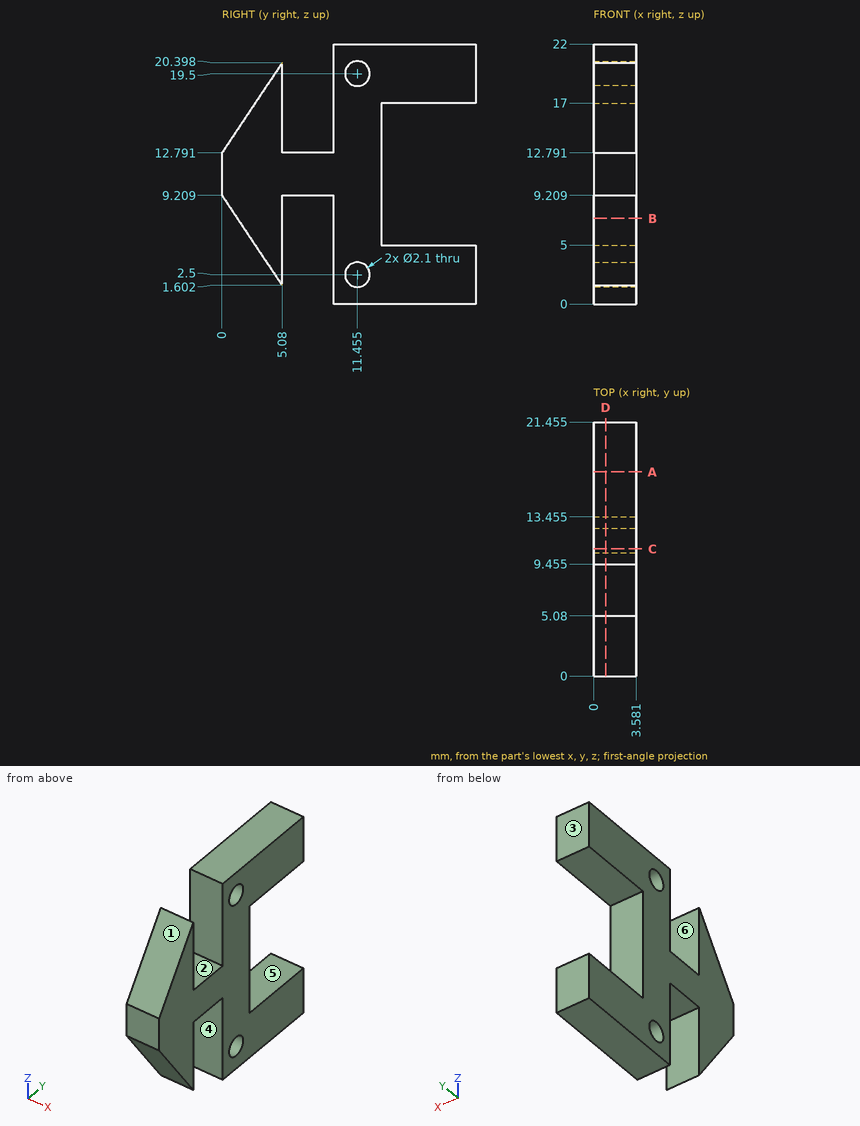
Answer from the drawing. Dimensions are ordinates in mm from the lowest x, y and z of the part. A direction names the side the tool comes from. Give positions to 0.01 mm unless a question says otherwise; leave off trailing zeros. Loops run counter-clockwise (first coordinate to the right, second up) from the corner with the lowest first, then second, coordinate; pieces in that order, holes last. Notation, with made-up numbers: (45.5, 52.25) -> (63.5, 52.25) arc R20 ccw to (63.5, 58.25) -> close; hole circle Ø4 at (-14.5, -32.5). An arc over 180 degrees is marked (long way). One line per question, with ' | ' between items. Start each with the question number.
1) Straight lines are drawn through the part: L1, parallel to Z at x = 1.45, y = 13.5; L2, parallel to Y at x = 1.75, z = 19.5 (1 decimal); L3, parallel to Z at x = 1.7, y = 5.75. For each, find the intervals that lie inside material, in ascending order.
2) Determine the mould class of the marked faces 1, 2 and 3 for opening direction Y: +Y half, -Y half, draft (parallel to the pull), parting line (faces both ways), or undercut.
3) Section B-B, the plane z = 7.25 is taken. Determine the outline of the cut face in (x, y) (1 decimal).
4) Section D-D, the plane x = 1 is taken. State how many separate pieces and enclosed holes the cut face has.
5) For the marked faces 4, 5 and 6, determine the directions among +Z, -Z, +X, -X, +Y, -Y from which every point of the face is accessible in a straight line to the end or side of a thin tool.
6) Section A-A, the plane y = 17.25 is taken. Determine the outline of the cut face in (x, z).
7) Each of these flat-tipped pins is pushed along its axis until it touches: pin 1 (2 mm diameter, centred on x = 2.5, z = 18, fed in from -Y); pin 2 (1.7 mm diameter, centred on y = 11.45, z = 2.5, fed in from -X); pin 3 (1.1 mm diameter, centred on x = 2, z = 12.5, fed in from +Y) (3 decimals); pin 4 (1.8 mm diameter, centred on x = 1.5, y = 7.5, fed in from +Z). Where does it stop, or does it pass through?
8) Section C-C, the plane y = 10.75 is taken. Determine the outline of the cut face in (x, z).
Resolved:
1) L1: 0 to 5, 17 to 22 | L2: 4.5 to 5.1, 9.5 to 10.4, 12.5 to 21.5 | L3: 9.21 to 12.79
2) face 1: -Y half | face 2: undercut | face 3: +Y half
3) outline: (0, 1.3) -> (3.6, 1.3) -> (3.6, 5.1) -> (0, 5.1) -> close; (0, 9.5) -> (3.6, 9.5) -> (3.6, 13.5) -> (0, 13.5) -> close
4) separate pieces: 1 | enclosed holes: 2
5) face 4: -Z, +X, -X | face 5: +X, -X, +Y | face 6: +Z, +X, -X
6) outline: (0, 0) -> (3.58, 0) -> (3.58, 5) -> (0, 5) -> close; (0, 17) -> (3.58, 17) -> (3.58, 22) -> (0, 22) -> close
7) pin 1: y = 2.81 | pin 2: through | pin 3: y = 13.455 | pin 4: z = 12.79
8) outline: (0, 0) -> (3.58, 0) -> (3.58, 1.72) -> (0, 1.72) -> close; (0, 3.28) -> (3.58, 3.28) -> (3.58, 18.72) -> (0, 18.72) -> close; (0, 20.28) -> (3.58, 20.28) -> (3.58, 22) -> (0, 22) -> close
